Source: CAD feature listing. Evaluate the final solid. Frame: model axes, mm. A direction names the side the tool comes from. Give positions to 0.01 mm unless a question says otherwise; leave off trailing zeros. Write each loop counter-clockwise with the first axis right and the second up, starting at its lowest first coordinate (ties: lowest second). Pieces come first, ordered by that corner, then holes. Notation, with made-up numbers: (-6, 33.5) -> (15, 33.5) arc R22 cw to (15, 40.5) -> close; hole circle Ø2 at (-10.75, 80). An arc over 180 degrees is marked (long way). Write item = value, one per line.
Autodesk Inventor part; units mm, degrees
ref_plane "YZ Plane" through (0, 0, 0) normal (1, 0, 0) x (0, 1, 0)
ref_plane "XZ Plane" through (0, 0, 0) normal (0, 1, 0) x (-1, 0, 0)
ref_plane "XY Plane" through (0, 0, 0) normal (0, 0, 1) x (1, 0, 0)
sketch "Sketch1" plane through (0, 0, 0) normal (0, 1, 0) x (-1, 0, 0)
  line L0 (-80, 27.5) -> (80, 27.5)
  line L1 (80, 27.5) -> (80, -27.5)
  line L2 (80, -27.5) -> (-80, -27.5)
  line L3 (-80, -27.5) -> (-80, 27.5)
  line L4 (-80, 27.5) -> (80, -27.5) construction
  line L5 (80, 27.5) -> (-80, -27.5) construction
  point P0 (0, 0)
  dimension "d0" = 160
  dimension "d1" = 55
extrude "Extrusion1" add sketch "Sketch1" along normal blind 4
sketch "Sketch2" plane through (0, 4, 0) normal (0, 1, 0) x (1, 0, 0)
  line L0 (80, 27.5) -> (-80, 27.5)
  line L1 (-80, 27.5) -> (-80, -27.5)
  line L2 (-80, -27.5) -> (80, -27.5)
  line L3 (80, -27.5) -> (80, 27.5)
  line L4 (-74, -23) -> (-9, -23)
  line L5 (-9, -23) -> (-9, 23)
  line L6 (-9, 23) -> (-74, 23)
  line L7 (-74, 23) -> (-74, -23)
  line L8 (-74, -23) -> (-74, -27.5)
  line L9 (-74, 23) -> (-74, 27.5)
  circle A0 centre (-74, -23) radius 1.55
  circle A1 centre (-74, 23) radius 1.55
  circle A2 centre (-9, -23) radius 1.55
  circle A3 centre (-9, 23) radius 1.55
  circle A4 centre (-74, 23) radius 5
  circle A5 centre (-9, 23) radius 5
  circle A6 centre (-74, -23) radius 5
  circle A7 centre (-9, -23) radius 5
  line L10 (-80, 0) -> (80, 0) construction
  line L11 (15.5, -13.25) -> (74, -13.25)
  line L12 (74, -13.25) -> (74, 13.25)
  line L13 (74, 13.25) -> (15.5, 13.25)
  line L14 (15.5, 13.25) -> (15.5, -13.25)
  line L15 (15.5, -13.25) -> (74, 13.25) construction
  line L16 (74, -13.25) -> (15.5, 13.25) construction
  circle A8 centre (15.5, -13.25) radius 2.05
  circle A9 centre (15.5, 13.25) radius 2.05
  circle A10 centre (74, 13.25) radius 2.05
  circle A11 centre (74, -13.25) radius 2.05
  circle A12 centre (15.5, 13.25) radius 4
  circle A13 centre (15.5, -13.25) radius 4
  circle A14 centre (74, -13.25) radius 4
  circle A15 centre (74, 13.25) radius 4
  point P0 (0, 0)
  point P1 (44.75, 0)
  point P2 (74, 9.25)
  point P3 (70, 13.25)
  point P4 (19.5, 13.25)
  point P5 (15.5, 9.25)
  point P6 (15.5, -9.25)
  point P7 (19.5, -13.25)
  point P8 (70, -13.25)
  point P9 (74, -9.25)
  point P10 (-14, -23)
  point P11 (-9, -18)
  point P12 (-9, 18)
  point P13 (-14, 23)
  point P14 (-69, 23)
  point P15 (-74, 18)
  point P16 (-74, -18)
  point P17 (-69, -23)
  dimension "d4" = 65
  dimension "d5" = 46
  dimension "d6" = 3.1
  dimension "d7" = 3.1
  dimension "d8" = 3.1
  dimension "d9" = 3.1
  dimension "d10" = 6
  dimension "d11" = 10
  dimension "d12" = 10
  dimension "d13" = 10
  dimension "d14" = 10
  dimension "d15" = 58.5
  dimension "d16" = 26.5
  dimension "d17" = 6
  dimension "d18" = 4.1
  dimension "d19" = 4.1
  dimension "d20" = 4.1
  dimension "d21" = 4.1
  dimension "d22" = 8
  dimension "d23" = 8
  dimension "d24" = 8
  dimension "d25" = 8
extrude "Extrusion2" cut sketch "Sketch2" against normal blind 10 contours A5 L5 A7 L4 A6 L7 A4 L6 | A3 L5 L6 | L6 L5 A3 | A1 L6 L9 | L9 L7 A1 | A1 L7 L6 | A2 L4 L5 | L5 L4 A2 | A0 L7 L8 | L8 L4 A0 | L4 L7 A0 | L14 A8 L11 | L11 A8 L14 | A13 L14 A12 L13 A15 L12 A14 L11 | A11 L12 L11 | L11 L12 A11 | A9 L13 L14 | L14 L13 A9 | A10 L13 L12 | L12 L13 A10
fillet "Fillet1" radius 2 4 edges at (-80, 2, 27.5) (80, 2, 27.5) (80, 2, -27.5) (-80, 2, -27.5)
sketch "Sketch3" plane through (0, 0, 0) normal (0, -1, 0) x (1, 0, 0)
  circle A0 centre (-9, 23) radius 1.55
  circle A1 centre (15.5, -13.25) radius 2.05
  circle A2 centre (-74, -23) radius 1.55
  circle A3 centre (74, -13.25) radius 2.05
  arc A4 (19.5, -13.25) -> (15.5, -9.25) centre (15.5, -13.25) ccw
  line L0 (15.5, -9.25) -> (15.5, 9.25)
  arc A5 (15.5, 9.25) -> (19.5, 13.25) centre (15.5, 13.25) ccw
  line L1 (19.5, 13.25) -> (70, 13.25)
  arc A6 (70, 13.25) -> (74, 9.25) centre (74, 13.25) ccw
  line L2 (74, 9.25) -> (74, -9.25)
  arc A7 (74, -9.25) -> (70, -13.25) centre (74, -13.25) ccw
  line L3 (70, -13.25) -> (19.5, -13.25)
  circle A8 centre (15.5, 13.25) radius 2.05
  circle A9 centre (-9, -23) radius 1.55
  circle A10 centre (-74, 23) radius 1.55
  circle A11 centre (74, 13.25) radius 2.05
  arc A12 (-9, -18) -> (-14, -23) centre (-9, -23) ccw
  line L4 (-14, -23) -> (-69, -23)
  arc A13 (-69, -23) -> (-74, -18) centre (-74, -23) ccw
  line L5 (-74, -18) -> (-74, 18)
  arc A14 (-74, 18) -> (-69, 23) centre (-74, 23) ccw
  line L6 (-69, 23) -> (-14, 23)
  arc A15 (-14, 23) -> (-9, 18) centre (-9, 23) ccw
  line L7 (-9, 18) -> (-9, -18)
  arc A16 (-80, -25.5) -> (-78, -27.5) centre (-78, -25.5) ccw
  line L8 (78, -27.5) -> (-78, -27.5)
  arc A17 (78, -27.5) -> (80, -25.5) centre (78, -25.5) ccw
  line L9 (80, 25.5) -> (80, -25.5)
  arc A18 (80, 25.5) -> (78, 27.5) centre (78, 25.5) ccw
  line L10 (-78, 27.5) -> (78, 27.5)
  arc A19 (-78, 27.5) -> (-80, 25.5) centre (-78, 25.5) ccw
  line L11 (-80, -25.5) -> (-80, 25.5)
  arc A20 (79.8, 25.5) -> (78, 27.3) centre (78, 25.5) ccw
  line L12 (79.8, 25.5) -> (79.8, -25.5)
  arc A21 (78, -27.3) -> (79.8, -25.5) centre (78, -25.5) ccw
  line L13 (78, -27.3) -> (-78, -27.3)
  arc A22 (-79.8, -25.5) -> (-78, -27.3) centre (-78, -25.5) ccw
  line L14 (-79.8, -25.5) -> (-79.8, 25.5)
  arc A23 (-78, 27.3) -> (-79.8, 25.5) centre (-78, 25.5) ccw
  line L15 (-78, 27.3) -> (78, 27.3)
  point P0 (0, 0)
  dimension "d29" = 0.2
extrude "offset" cut sketch "Sketch3" against normal through all contours L11 A19 L10 A18 L9 A17 L8 A16
properties part number "motherboard"
1) Material intervals for L1, parallel to X at y = 0.5, z = 0; L2, parallel to Z at x = 60, y = 3.4; L3, parallel to X at y = 2.6, z = 14, sorted ascending.
Computed:
L1 = -79.8 to -74, -9 to 15.5, 74 to 79.8
L2 = -27.3 to -13.25, 13.25 to 27.3
L3 = -79.8 to -74, -9 to 13.59, 17.41 to 72.09, 75.91 to 79.8
2) Access query for faces 4 (the flat face through (19, 0, 13)), 5 (the cylindrical face through (-71, 2, -19)). Directions: +Z, -Z, +X, -X, +Y, -Y. A direction counts if a zero-diameter tool reaches every point of the face in a straight line with its end or side. Return the directions, or none.
Computed:
face_4 = +Z, -Z, +X, -X, -Y
face_5 = +Y, -Y
3) Draft query along X for faces 1 (the flat face through (19, 4, 13)), 2 (the cylindrical face through (-70, 2, 20)), 3 (the flat face through (-79.8, 2, 0)). Return one class per face: pulls with the +X half, pulls with the -X half, needs draft (parallel to the pull), parting line crosses it, or undercut.
Computed:
face_1 = needs draft
face_2 = undercut
face_3 = pulls with the -X half
4) Cut plane C-C (z = 1.5). Return the cut outline in (x, y), then the cut area to 3 significant figures.
Computed:
outline = (-79.8, 0) -> (-74, 0) -> (-74, 4) -> (-79.8, 4) -> close; (-9, 0) -> (15.5, 0) -> (15.5, 4) -> (-9, 4) -> close; (74, 0) -> (79.8, 0) -> (79.8, 4) -> (74, 4) -> close
area = 144 mm²
5) Cut plane A-A (x = 48). Return the cut outline in (y, z).
Computed:
outline = (0, -27.3) -> (4, -27.3) -> (4, -13.25) -> (0, -13.25) -> close; (0, 13.25) -> (4, 13.25) -> (4, 27.3) -> (0, 27.3) -> close
6) Cut plane B-B (y = 3.15). State how many separate pieces and enclosed holes the cut face has, then the cut area to 3 significant figures.
Computed:
separate_pieces = 1
enclosed_holes = 10
area = 4,220 mm²
